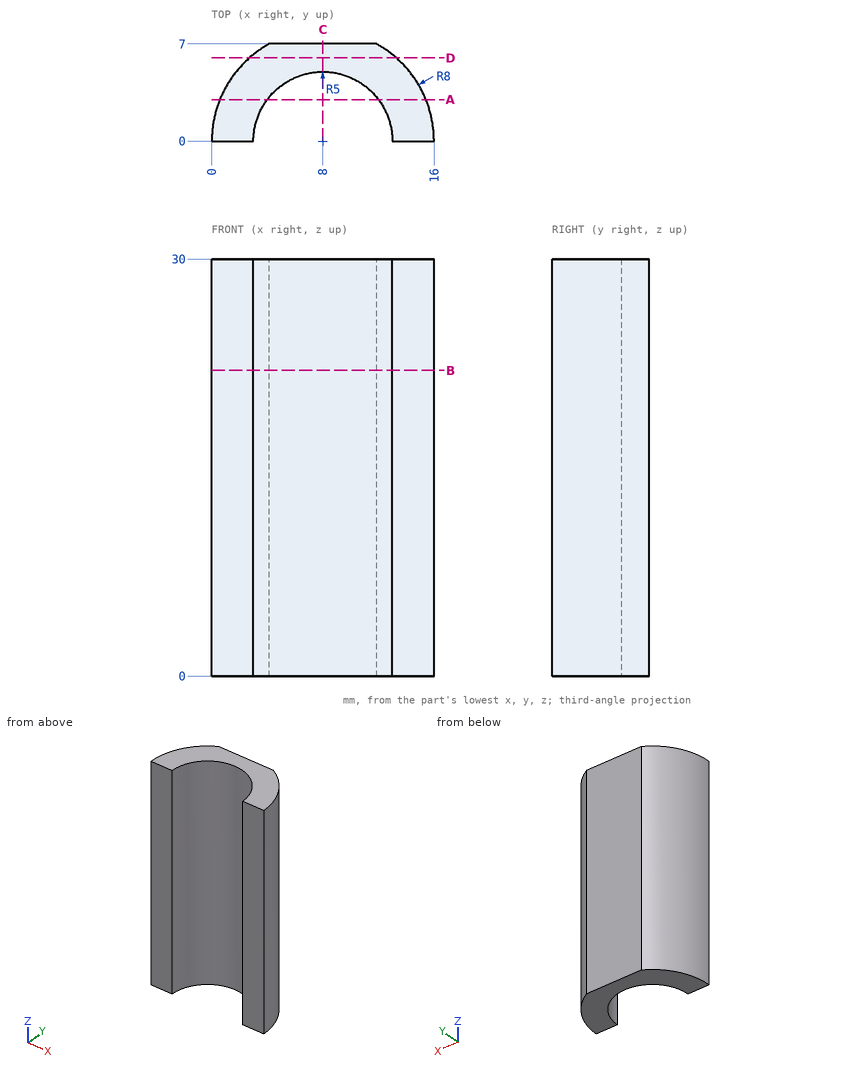
Can you work these out from the drawing? Everything is in mm from the part's minimum corner. Round coordinates to 2 decimals unless told otherwise and drop trailing zeros. Order: outer loops, then holes, each group sorted by start corner. A loop starts at its lowest first (then second) coordinate and runs counter-clockwise, first axis right, second up. Notation, with made-up numbers: (-25.75, 83.25) - (1.25, 83.25) arc R35 cw to (1.25, 119.25) - close; hole circle Ø1 at (-4.5, 44). An arc over 180 degrees is marked (long way). Answer in a Markdown table with one row per item.
(1) Suppose I cut it at B-B, the plane z = 22. Please give me the cut outline in (x, y).
From the geometry:
| item | result |
|---|---|
| outline | (0, 0) - (3, 0) arc R5 cw to (13, 0) - (16, 0) arc R8 ccw to (11.87, 7) - (4.13, 7) arc R8 ccw to start |
(2) Suppose I cut it at D-D, the plane y = 6. Please give me the cut outline in (x, z).
From the geometry:
| item | result |
|---|---|
| outline | (2.71, 0) - (13.29, 0) - (13.29, 30) - (2.71, 30) - close |
(3) For P1, Ø2, axis at y = 5.5, z = 10, coming from the -X side, with a flat end and sliding along its axis, tell me the tip position at first contact or that it passes through.
From the geometry:
| item | result |
|---|---|
| P1 | stops at x = 1.39 |
(4) Suppose I cut it at A-A, the plane y = 3. Please give me the cut outline in (x, z), plus the area to 3 significant figures.
From the geometry:
| item | result |
|---|---|
| outline | (0.58, 0) - (4, 0) - (4, 30) - (0.58, 30) - close; (12, 0) - (15.42, 0) - (15.42, 30) - (12, 30) - close |
| area | 205 mm2 |
(5) Please list where these lines run through material, in increasing order: L1, parallel to X at y = 1.5, z = 27.75; L2, parallel to X at y = 3.75, z = 15.5; L3, parallel to Y at x = 5.25, z = 24.5. Write a range as from..to.
From the geometry:
| item | result |
|---|---|
| L1 | x = 0.14..3.23, 12.77..15.86 |
| L2 | x = 0.93..4.69, 11.31..15.07 |
| L3 | y = 4.18..7 |
(6) Suppose I cut it at C-C, the plane x = 8. Please give me the cut outline in (y, z).
From the geometry:
| item | result |
|---|---|
| outline | (5, 0) - (7, 0) - (7, 30) - (5, 30) - close |
